Design review of the part shown in the three views and the two pictorial views. Dimensions are in mm from the part's minimum x, y and z. Give positions to 0.01 mm unless a question says otherwise; leave off trailing zeros. Loops run counter-clockwise (first coordinate to the right, second up) from the corner with the lowest first, then second, coordinate; pieces in that order, holes last. Notation, with made-up numbers: (-5, -22) - (40, -22) arc R15 ccw to (40, -8) - close; hole circle Ø7 at (17, -30.5). An arc over 180 degrees is marked (long way). Answer as a JSON object with one key per item and string values.
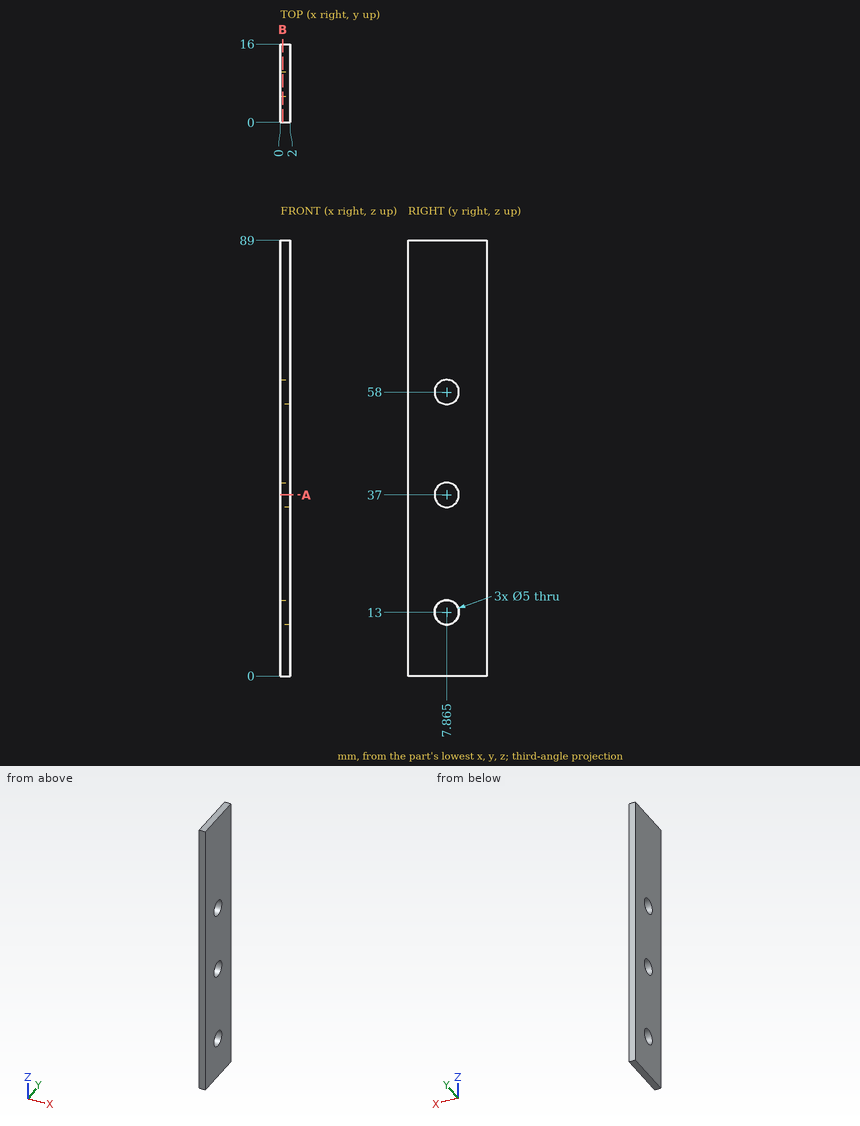
Q1. To check wall thickness, follow probe 1 along Z at (x, y) = (0.65, 7.75); probe 2 along Y at (x, z) = (0.6, 37) (1 decimal); probe 3 along Z at (x, y) = (1.95, 6.5) (1 decimal). State the ranges of each line that lie inside material, in increasing order. Write a range as [from, to].
Results:
{"probe 1": "z = [0, 10.5], [15.5, 34.5], [39.5, 55.5], [60.5, 89]", "probe 2": "y = [0, 5.4], [10.4, 16]", "probe 3": "z = [0, 10.9], [15.1, 34.9], [39.1, 55.9], [60.1, 89]"}
Q2. Consider section B-B, the plane x = 0.45. State the section outline as (y, z) points (1 decimal), plus the area to 4 significant figures.
Results:
{"outline": "(0, 0) - (16, 0) - (16, 89) - (0, 89) - close; hole circle Ø5 at (7.9, 13); hole circle Ø5 at (7.9, 37); hole circle Ø5 at (7.9, 58)", "area": "1,365 mm^2"}
Q3. Consider section A-A, the plane z = 37. State the section outline as (x, y) points (1 decimal).
Results:
{"outline": "(0, 0) - (2, 0) - (2, 5.4) - (0, 5.4) - close; (0, 10.4) - (2, 10.4) - (2, 16) - (0, 16) - close"}
